Answer from the drawing. Dimensions are ordinates in mm from the lowest x, y and z of the part. Coordinates: 2 decimals unless noted, no trailing zeros. Loops run counter-clockwise (first coordinate to the right, second up) from the corner with the lowest first, then second, coordinate; pieces in that order, holes last. Notation, with made-up numbers: (-20, 63.25) -> (11, 63.25) arc R26 ccw to (11, 87.25) -> close; hole circle Ø8 at (63, 64.5). An arc over 180 degrees is marked (long way). Use a Markdown table: item, result.
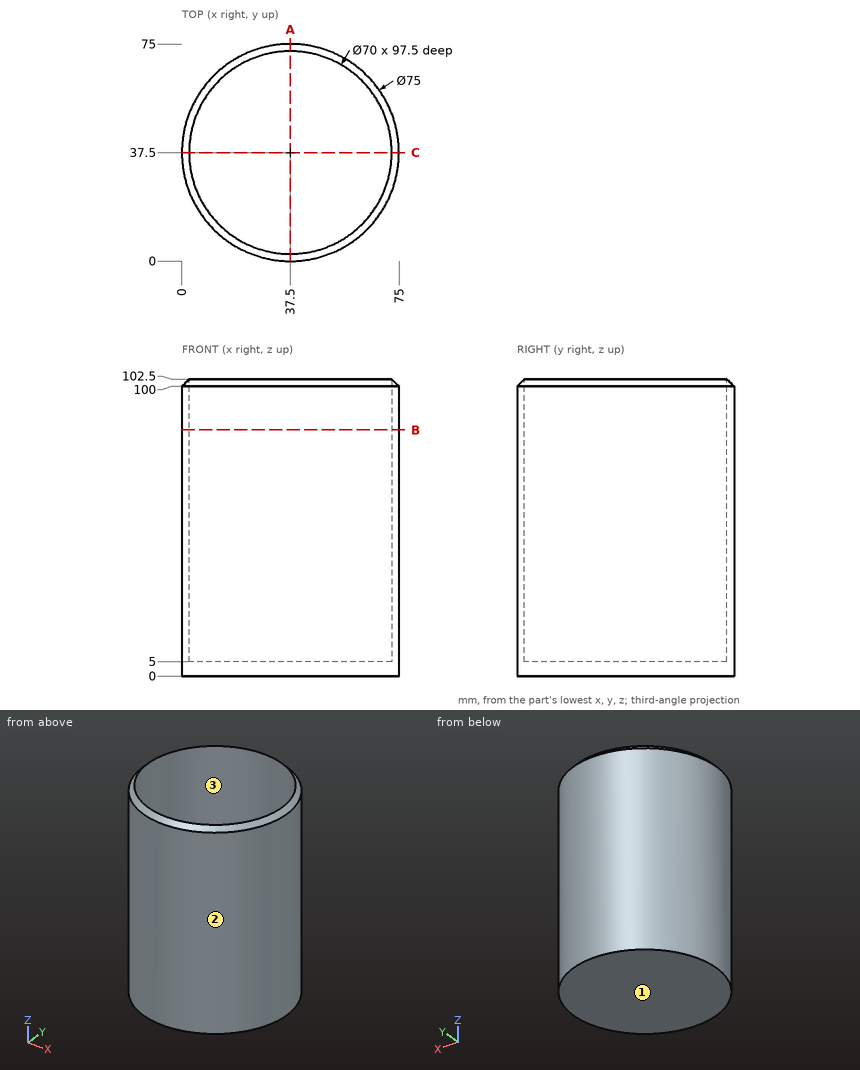
Q1. Determine the mould class of the marked faces 1, 2 and 3 for opening direction Y: pulls with the +Y half, pulls with the -Y half, needs draft (parallel to the pull), parting line crosses it, or undercut.
Solved:
| item | result |
|---|---|
| face 1 | needs draft |
| face 2 | parting line crosses it |
| face 3 | undercut |
Q2. Consider line 1 (Y direction, x = 37.5, z = 39.5); line 2 (Z direction, x = 13.5, y = 30). Determine where each line is inside the solid, lowest interval first. Write a range as [from, to].
Solved:
| item | result |
|---|---|
| line 1 | [0, 2.5], [72.5, 75] |
| line 2 | [0, 5] |
Q3. Given pin 1 Ø10 at (x, z) = (10, 42) entering from -Y; pin 2 Ø1 at (x, y) = (21.5, 17) entering from -Z; pin 3 Ø2 at (y, z) = (17.5, 34) entering from -X; pin 4 Ø1 at (x, z) = (60, 20) entering from -Y, each flat-ended and moving along its own axis, determine where each tip first touches the part or whether it passes through.
Solved:
| item | result |
|---|---|
| pin 1 | y = 7.5 |
| pin 2 | z = 0 |
| pin 3 | x = 5.17 |
| pin 4 | y = 7.13 |
Q4. Section A-A on x = 37.5 is taken. Determine the outline of the cut face in (y, z), and give its area (3 significant figures).
Solved:
| item | result |
|---|---|
| outline | (0, 0) -> (75, 0) -> (75, 100) -> (72.5, 102.5) -> (72.5, 5) -> (2.5, 5) -> (2.5, 102.5) -> (0, 100) -> close |
| area | 856 mm² |
Q5. Section B-B on z = 85 is taken. Determine the outline of the cut face in (x, y).
Solved:
| item | result |
|---|---|
| outline | circle Ø75 at (37.5, 37.5); hole circle Ø70 at (37.5, 37.5) |
